Verification items for the finished model (mm, model axes). Round coordinates to 2 decimals unless told otherwise and drop trailing zeros. Loops run counter-clockwise (first coordinate to the right, second up) from the corner with the lowest first, then second, coordinate; pieces in that order, holes last.
from build123d import *

# Parameters (mm, degrees)
AUFSATZ_LINEAR_AUSTRAGEN1_DEPTH = 2


with BuildPart() as part:
    # Skizze1 → Aufsatz-Linear austragen1 (new body)
    with BuildSketch(Plane(origin=(0, 0, 0), x_dir=(1, 0, 0), z_dir=(0, 1, 0))):
        with BuildLine():
            Line((-111.014713036, 96.629952772), (-111.014713036, 82.637944818))
            ThreePointArc((-111.014713036, 82.637944818), (-133.773093964, 70.056299779), (-155.121581381, 55.20760356))
            Line((-155.121581381, 55.20760356), (-176.68443544, 58.018627787))
            Line((-176.68443544, 58.018627787), (-184.391490567, 48.817347687))
            ThreePointArc((-184.391490567, 48.817347687), (-184.856553748, 45.106419523), (-183.300343728, 41.705613446))
            Line((-183.300343728, 41.705613446), (-179.406379638, 37.139090384))
            Line((-179.406379638, 37.139090384), (-183.244712688, 33.192915196))
            Line((-183.244712688, 33.192915196), (-181.577621487, 31.571382711))
            ThreePointArc((-181.577621487, 31.571382711), (-234.688503419, -49.730678526), (-253.304201651, -145.041993281))
            Line((-253.304201651, -145.041993281), (253.3, -145.041993281))
            ThreePointArc((253.3, -145.041993281), (213.679953091, -9.020178425), (107.2140887, 84.450148167))
            Line((107.2140887, 84.450148167), (88.10582283, 137.079482634))
            ThreePointArc((88.10582283, 137.079482634), (83.551519794, 142.896881485), (76.497849408, 145.094502845))
            Line((76.497849408, 145.094502845), (73.732714296, 145.093801448))
            add(Edge.make_bspline(
                [(61.241798353, 137.079482633), (63.12872124, 142.063691586), (68.556952847, 144.691016446), (73.732714296, 145.093801449)],
                knots=[0, 0, 0, 0, 0.846643391, 0.846643391, 0.846643391, 0.846643391], degree=3))
            Line((61.241798353, 137.079482633), (49.403316926, 103.395240199))
            ThreePointArc((49.403316926, 103.395240199), (47.136635501, 103.835273299), (44.866037129, 104.254626189))
            Line((44.866037129, 104.254626189), (44.866037129, 145.086479208))
            Line((44.866037129, 145.086479208), (8.335497246, 145.077212974))
            Line((8.335497246, 145.077212974), (6.400480376, 145.076722143))
            add(Edge.make_bspline(
                [(-9.859797389, 131.748243103), (-9.468785698, 135.744179636), (-3.989815347, 141.108587237), (2.485358217, 144.80702629), (6.400480376, 145.076722143)],
                knots=[0, 0, 0, 0, 0.454488203, 0.924546926, 0.924546926, 0.924546926, 0.924546926], degree=3))
            Line((-9.859797389, 131.748243103), (-9.859797389, 145.072597607))
            Line((-9.859797389, 145.072597607), (-38.85877651, 145.065241807))
            add(Edge.make_bspline(
                [(-59.546942015, 131.748243103), (-56.872959995, 140.401818923), (-47.428583468, 145.063068014), (-38.85877651, 145.065241807)],
                knots=[0, 0, 0, 0, 1, 1, 1, 1], degree=3))
            Line((-59.546942015, 131.748243103), (-59.546942015, 145.059994105))
            Line((-59.546942015, 145.059994105), (-87.539763433, 145.052893525))
            add(Edge.make_bspline(
                [(-97.500864535, 96.629952772), (-104.579533848, 99.859372788), (-116.831393377, 118.836705983), (-105.084694212, 143.726198357), (-87.539763433, 145.052893525)],
                knots=[0, 0, 0, 0, 0.332503248, 1, 1, 1, 1], degree=3))
            Line((-97.500864535, 96.629952772), (-111.014713036, 96.629952772))
        make_face()
    extrude(amount=AUFSATZ_LINEAR_AUSTRAGEN1_DEPTH)


solid = part.part
1. Release check for a two-part mould opening along X. For faces 1 (the face through (97.794, 0.986, -110.396)), 2 (the face through (-4, 0, 30)), 3 (the face through (-234.17, 0.99, 48.46)), 4 (the face through (55.405, 0.986, -120.473)) record: released by +X, released by -X, zero draft, split by the parting line, or undercut.
2. Section check B-B (x = -117.5). Enter the section's corners in (y, z), then the cut area to 3 significant figures.
3. Gauge pin test, flat ends, axial feed: P1, Ø0.6, axis at x = -103, y = 1, coming from the -Z side; P2, Ø0.6, axis at x = -73, y = 0.5, coming from the -Z side; P3, Ø1, axis at y = 0.5, z = -113, coming from the -X side. Record the tip position at first contact, or that the pin passes through.
4. Scan lines: L1, parallel to Z at x = -26.5, y = 1.45; L2, parallel to Z at x = 211.5, y = 0.95; L3, parallel to X at y = 0.4, z = 98. Record each from-to range of solid material in increasing order.
5. Section check A-A (z = -66.5). Enter the section's corners in (x, y).
Taken from the geometry:
1. face 1: released by +X
1. face 2: zero draft
1. face 3: released by -X
1. face 4: undercut
2. outline: (0, -79.36) - (2, -79.36) - (2, 145.04) - (0, 145.04) - close
2. area: 449 mm2
3. P1: stops at z = -138.48
3. P2: stops at z = -145.06
3. P3: stops at x = -110.15
4. L1: z = -145.07 to 145.04
4. L2: z = 5.65 to 145.04
4. L3: x = -248.9 to 248.89
5. outline: (-139.33, 0) - (139.32, 0) - (139.32, 2) - (-139.33, 2) - close
